Geometry check sheet. Reference: the model listing, model coordinates, mm. A direction names the side the tool comes from. Round coordinates to 2 decimals unless told otherwise and drop trailing zeros. Order: outer loops, then holes, each group sorted by start corner. A loop starts at its lowest first (then second) coordinate and runs counter-clockwise, first axis right, second up. Notation, with made-up numbers: M 38.5,40 L 74.5,40 A7 cw 74.5,46 Z; hole C 56,22 d1. An arc over 180 degrees is marked long. Answer as a JSON object with one key per item and string values. Group by question number.
```python
from build123d import *

# Parameters (mm, degrees)
ESBO_O1_W               = 56
ESBO_O1_H               = 12.7
FLANGE_BASE1_DEPTH      = 3.18
DOBRA_START             = -6.35
DOBRA_ESBO_ADA1_DEPTH   = 12.7
DOBRA_ESBO_ADA1_2_DEPTH = 12.7
ESBO_O7_R               = 2.75
CORTE_EXTRUS_O2_DEPTH   = 10
ESBO_O11_R              = 1.65
CORTE_EXTRUS_O3_DEPTH   = 10


# Read off the part's stored shape, not the designer's step: Dobra esboçada1
# Sheet-metal steps are written as plain solids
with BuildPart() as part:
    # Esboço1 → Flange-base1 (new body)
    with BuildSketch(Plane.XY):
        Rectangle(ESBO_O1_W, ESBO_O1_H)
    extrude(amount=-FLANGE_BASE1_DEPTH)

    # Dobra esboçada1 outline → Dobra esboçada1 (cut)
    with BuildSketch(Plane(origin=(0, 0, 0), x_dir=(1, 0, 0), z_dir=(0, 1, 0)).offset(DOBRA_START)):
        with BuildLine():
            ThreePointArc((0.50243384, 3.18), (3.68243384, 2.327921568), (6.010355408, 0))
            Line((6.010355408, 0), (28, 0))
            Line((28, 0), (28, 3.18))
            Line((28, 3.18), (0.50243384, 3.18))
        make_face()
    extrude(amount=DOBRA_ESBO_ADA1_DEPTH, mode=Mode.SUBTRACT)

    # Dobra esbo_ada1 2 outline → Dobra esbo_ada1 2 (add)
    with BuildSketch(Plane(origin=(0, 0, 0), x_dir=(1, 0, 0), z_dir=(0, 1, 0)).offset(DOBRA_START)):
        with BuildLine():
            Line((3.256394624, -1.59), (14.507611545, -21.077679353))
            Line((14.507611545, -21.077679353), (17.261572329, -19.487679353))
            Line((17.261572329, -19.487679353), (6.010355408, 0))
            Line((6.010355408, 0), (0.50243384, 0))
            ThreePointArc((0.50243384, 0), (2.09243384, -0.426039216), (3.256394624, -1.59))
        make_face()
    extrude(amount=DOBRA_ESBO_ADA1_2_DEPTH)

    # Esboço7 → Corte-extrusão2 (cut)
    with BuildSketch(Plane(origin=(0, 0, -3.18), x_dir=(-1, 0, 0), z_dir=(0, 0, -1))):
        with Locations((12.150906248, 0)):
            Circle(ESBO_O7_R)
    extrude(amount=-CORTE_EXTRUS_O2_DEPTH, mode=Mode.SUBTRACT)

    # Esboço11 → Corte-extrusão3 (cut)
    with BuildSketch(Plane(origin=(1.753805772, 0, -1.012560235), x_dir=(0.49999999999999806, 0, 0.8660254037844398), z_dir=(-0.8660254037844397, 0, 0.499999999999998))):
        with Locations((18.257611545, -0.33)):
            Circle(ESBO_O11_R)
    extrude(amount=-CORTE_EXTRUS_O3_DEPTH, mode=Mode.SUBTRACT)


solid = part.part
```
1) Sectioned sample at C-C (y = -1.25). Record the boundary of the cut face in (x, z).
2) Sectioned sample at A-A (y = -4). Record the boundary of the cut face in (x, z), then the cut area to 3 significant figures.
3) Thickness scan on line 1 along Z through (x, y) = (-19.5, -4.75); line 2 along X through (y, z) = (2.5, 17); line 3 along Z through (x, y) = (13.5, -1). Record the ranges inside material, lowest first. Write a range as [from, to].
4) Sectioned sample at B-B (x = -13.5). Record the boundary of the cut face in (y, z).
5) Set-up check for faces 1 (the flat face through (-5, -6.35, -1)), 2 (the flat face through (-14, -3, 0)): record each of +Z, -Z, +X, -X, +Y, -Y from which the full face is reachable in a straight line by a thin tool's end or side.
6) Sectioned sample at D-D (z = 8.5). Record the boundary of the cut face in (x, y), then the cut area to 3 significant figures.
7) Release check for a two-part mould opening along X. For faces 3 (the cylindrical face through (13.002, -0.962, 15.335)), 4 (the flat face through (8.803, -0.089, 11.197)), 5 (the flat face through (11.715, -0.089, 9.88)) record: +X half, -X half, draft (parallel to the pull), parting line (faces both ways), or undercut.
8) Go/stop test with flat-tipped pins: P1, Ø3, axis at y = 1.5, z = 5.5, coming from the +X side; P2, Ø3, axis at y = -1.5, z = 8.5, coming from the +X side; P3, Ø6, axis at x = -11, y = -3.5, coming from the +Z side. Record where each tip stops, or that it passes through.
Final values:
{
 "1": {"outline": "M -28,-3.18 L -14.6,-3.18 L -14.6,0 L -28,0 Z; M -9.7,-3.18 L 0.5,-3.18 A6.36 ccw 6.01,0 L 12.95,12.02 L 10.2,13.61 L 3.26,1.59 A3.18 cw 0.5,0 L -9.7,0 Z; M 11.57,15.99 L 14.32,14.4 L 17.26,19.49 L 14.51,21.08 Z"},
 "2": {"outline": "M -28,-3.18 L 0.5,-3.18 A6.36 ccw 6.01,0 L 17.26,19.49 L 14.51,21.08 L 3.26,1.59 A3.18 cw 0.5,0 L -28,0 Z", "area": "178 mm^2"},
 "3": {"line 1": "z = [-3.18, 0]", "line 2": "x = [12.15, 15.83]", "line 3": "z = [15.03, 19.33]"},
 "4": {"outline": "M -6.35,-3.18 L -2.4,-3.18 L -2.4,0 L -6.35,0 Z; M 2.4,-3.18 L 6.35,-3.18 L 6.35,0 L 2.4,0 Z"},
 "5": {"face 1": "+Z, -Z, +X, -X, -Y", "face 2": "+Z, -X, +Y, -Y"},
 "6": {"outline": "M 7.25,-6.35 L 10.92,-6.35 L 10.92,6.35 L 7.25,6.35 Z", "area": "46.6 mm^2"},
 "7": {"face 3": "undercut", "face 4": "-X half", "face 5": "+X half"},
 "8": {"P1": "stops at x = 10.05", "P2": "stops at x = 11.78", "P3": "stops at z = 0"}
}
